```python
from build123d import *

# Parameters (mm, degrees)
F0_W     = 342.9
F0_H     = 203.2
F1_DEPTH = 355.6
F6_W     = 76.2
F6_H     = 38.1
F7_DEPTH = 25.4


# Not quite as in the source:
# - a pattern or mirror of a feature is missing from the dataset's text; its kind, count and spacing are read off the source's solid


with BuildPart() as f1:
    # F0 (on Top) → F1 (new body)
    with BuildSketch(Plane.XY):
        with Locations((171.45, 101.6)):
            Rectangle(F0_W, F0_H)
    extrude(amount=F1_DEPTH)

    # F3 (on offset) → F4 (revolve)
    with BuildSketch(Plane.XZ.offset(-50.8)):
        with BuildLine():
            Line((63.5, 381), (63.5, 355.6))
            Line((63.5, 355.6), (85.725, 355.6))
            Line((85.725, 355.6), (85.725, 361.95))
            ThreePointArc((85.725, 361.95), (83.8651280605, 366.4401280605), (79.375, 368.3))
            Line((79.375, 368.3), (74.6125, 368.3))
            ThreePointArc((74.6125, 368.3), (72.7526280605, 372.7901280605), (68.2625, 374.65))
            Line((68.2625, 374.65), (68.2625, 381))
            Line((68.2625, 381), (63.5, 381))
        make_face()
    f4 = revolve(axis=Axis((63.5, 50.8, 362.4166101217), (0, 0, 1)))

    # F4_copies: F4 across plane
    add(f4.mirror(Plane(origin=(171.45, 0, 0), x_dir=(0, 0, 1), z_dir=(1, 0, 0))))

    # F6 (on face) → F7 (cut)
    with BuildSketch(Plane(origin=(0, 0, 0), x_dir=(0, -1, 0), z_dir=(-1, 0, 0))):
        with Locations((-101.6, 298.45)):
            Rectangle(F6_W, F6_H)
    f7 = extrude(amount=-F7_DEPTH, mode=Mode.SUBTRACT)

    # F7_copies: F7 across plane
    add(f7.mirror(Plane(origin=(171.45, 0, 0), x_dir=(0, 0, 1), z_dir=(1, 0, 0))), mode=Mode.SUBTRACT)


solid = f1.part
```
Verification items for the finished model (mm, model axes). A direction names the side the tool comes from. Round coordinates to 2 decimals unless told otherwise and drop trailing zeros. Order: outer loops, then holes, each group sorted by start corner. A loop starts at its lowest first (then second) coordinate and runs counter-clockwise, first axis right, second up. Notation, with made-up numbers: (63.25, -4.75) -> (116.25, -4.75) arc R15 cw to (116.25, 1.25) -> close; hole circle Ø4 at (85.25, 77). An arc over 180 degrees is marked (long way). Put each result on its own line as item: value. Start each with the question number.
(1) Tool access check on faces 1 (the face through (13, 139.7, 298)), 2 (the face through (84.699, 57.476, 358.819)), 3 (the face through (330, 102, 317.5)). Record the directions out of +Z, -Z, +X, -X, +Y, -Y that give a thin tool (end or side, any length) a straight path to the whole face; none if there is none.
(2) Section check A-A (y = 78). Enter the section's corners in (x, z).
(3) Section check C-C (y = 174). Enter the section's corners in (x, z).
(4) Material ranges on line 1 along Z through (x, y) = (43.5, 20); line 2 along X through (y, z) = (137, 291.5); line 3 along Z through (x, y) = (281.5, 42), recorded low to high.
(5) Draft check along Y on faces 4 (the face through (13, 63.5, 298)), 5 (the face through (258.201, 57.476, 358.819)), 6 (the face through (13, 102, 317.5)), 7 (the face through (290.2, 47.5, 368.3)). Enter one of: +Y half, -Y half, draft (parallel to the pull), parting line (faces both ways), or undercut.
(6) Depth check by flat-ended pin: pin 1 Ø10 at (x, y) = (246, 45) entering from +Z; pin 2 Ø11.5 at (y, z) = (90.5, 291) entering from -X. Enter the tip coordinate at first touch or a pass-through.
(7) Section check B-B (x = 192). Enter the section's corners in (y, z).
Completed:
1. face 1: -X
1. face 2: +Z
1. face 3: +X
2. outline: (0, 0) -> (342.9, 0) -> (342.9, 279.4) -> (317.5, 279.4) -> (317.5, 317.5) -> (342.9, 317.5) -> (342.9, 355.6) -> (0, 355.6) -> (0, 317.5) -> (25.4, 317.5) -> (25.4, 279.4) -> (0, 279.4) -> close
3. outline: (0, 0) -> (342.9, 0) -> (342.9, 355.6) -> (0, 355.6) -> close
4. line 1: z = 0 to 355.6
4. line 2: x = 25.4 to 317.5
4. line 3: z = 0 to 372.99
5. face 4: undercut
5. face 5: parting line
5. face 6: undercut
5. face 7: draft
6. pin 1: stops at z = 355.6
6. pin 2: stops at x = 25.4
7. outline: (0, 0) -> (203.2, 0) -> (203.2, 355.6) -> (0, 355.6) -> close
